Design review of the part built by this model. Coordinates are the model's own, in mm. A direction names the side the tool comes from. Coordinates: 2 decimals unless noted, no trailing zeros. Write each loop counter-clockwise with the first axis right and the second up, starting at its lowest first coordinate (ties: lowest second). Pieces come first, ordered by that corner, then holes. Notation, with made-up numbers: (21, 9.5) -> (29, 9.5) arc R24 ccw to (29, 20.5) -> close; hole circle Ø1 at (56.5, 6). An arc over 180 degrees is marked (long way). Answer in a Markdown table with one row per item. Add a question column.
Item 1: Take a section at B-B, the plane x = 194.5. Write out the cut boundary in (y, z) (1 decimal), and give its area (3 significant figures).
Item 2: Take a section at A-A, the plane z = 155. Write out the cut boundary in (x, y) (1 decimal).
Item 3: Draft analysis for pull direction X (two halves, no side actions). For faces 1 (the face through (-3, 0, -49)), 2 (the face through (-229.69, -4.83, 158.36)), state which applies: released by +X, released by -X, zero draft, split by the parting line, or undercut.
Item 4: To check wall thickness, follow line 1 (Z direction, x = 29, y = -7.5); line 2 (X direction, y = -5.75, z = 153); line 3 (Z direction, x = -192.5, y = -4). State the ranges of each line that lie inside material, in increasing order.
Item 5: For faces 3 (the face through (229.69, -4.83, 155.97)), 4 (the face through (-3, -9.525, -49)), list the 3-axis set-ups (+Z, -Z, +X, -X, +Y, -Y) from which the entire face can be reached by the end or side of a thin tool; tool diameter is ignored.
Item 6: Take a section at C-C, the plane y = -4.5. Write out the cut boundary in (x, z), and give its area (3 significant figures).
from build123d import *

# Parameters (mm, degrees)
F0_W     = 485.775
F0_H     = 473.075
F1_DEPTH = 9.525
F3_D     = 109.982
F4_DEPTH = 25.4


with BuildPart() as f1:
    # F0 (on Front) → F1 (new body)
    with BuildSketch(Plane.XZ):
        Rectangle(F0_W, F0_H)
    extrude(amount=F1_DEPTH)

    # F3 (through all)
    with Locations(Plane.XZ.offset(9.525)):
        with Locations((0, 157.1625)):
            Hole(F3_D / 2)

    # F2 (on face) → F4 (cut)
    with BuildSketch(Plane.XZ.offset(9.525)):
        with BuildLine():
            Line((-152.444478, 226.1625), (-187.189204, 226.1625))
            ThreePointArc((-187.189204, 226.1625), (-229.698578, 157.1625), (-187.189204, 88.1625))
            Line((-187.189204, 88.1625), (-152.444478, 88.1625))
            Line((-152.444478, 88.1625), (152.444478, 88.1625))
            Line((152.444478, 88.1625), (187.189204, 88.1625))
            ThreePointArc((187.189204, 88.1625), (229.698578, 157.1625), (187.189204, 226.1625))
            Line((187.189204, 226.1625), (152.444478, 226.1625))
            Line((152.444478, 226.1625), (-152.444478, 226.1625))
        make_face()
    extrude(amount=-F4_DEPTH, mode=Mode.SUBTRACT)


solid = f1.part
Answers:
| question | item | result |
|---|---|---|
| 1 | outline | (-9.5, -236.5) -> (0, -236.5) -> (0, 92.4) -> (-9.5, 92.4) -> close; (-9.5, 222) -> (0, 222) -> (0, 236.5) -> (-9.5, 236.5) -> close |
| 1 | area | 3,270 mm^2 |
| 2 | outline | (-242.9, -9.5) -> (-229.7, -9.5) -> (-229.7, 0) -> (-242.9, 0) -> close; (229.7, -9.5) -> (242.9, -9.5) -> (242.9, 0) -> (229.7, 0) -> close |
| 3 | face 1 | zero draft |
| 3 | face 2 | undercut |
| 4 | line 1 | z = -236.54 to 88.16, 226.16 to 236.54 |
| 4 | line 2 | x = -242.89 to -229.59, 229.59 to 242.89 |
| 4 | line 3 | z = -236.54 to 91.1, 223.22 to 236.54 |
| 5 | face 3 | +Y, -Y |
| 5 | face 4 | +Z, -Z, +X, -X, -Y |
| 6 | outline | (-242.89, -236.54) -> (242.89, -236.54) -> (242.89, 236.54) -> (-242.89, 236.54) -> close; hole (-187.19, 88.16) -> (187.19, 88.16) arc R77.25 ccw to (187.19, 226.16) -> (-187.19, 226.16) arc R77.25 ccw to start |
| 6 | area | 170,000 mm^2 |
